CAD build for the part. Positions are in the model's coordinates, mm. Round coordinates to 2 decimals unless told otherwise and drop trailing zeros. Order: outer loops, then holes, each group sorted by start corner. A loop starts at its lowest first (then second) coordinate and runs counter-clockwise, first axis right, second up. Notation, with made-up numbers: M 76.5,15.25 L 83.5,15.25 A28 ccw 83.5,36.25 Z; hole C -30.5,-13 d3. An arc over 180 degrees is marked long. Put each result on its own line as item: value.
```python
from build123d import *

# Parameters (mm, degrees)
SKETCH_1_W                 = 10.16
SKETCH_1_H                 = 2.5
EXTRUDE_1_DEPTH            = 2.5
EXTRUDE_START              = -5
SKETCH_2_R                 = 0.3
EXTRUDE_2_DEPTH            = 7.5
PATTERN_LINEAR_1_COUNT     = 3
PATTERN_LINEAR_1_PITCH     = 2.54
PATTERN_LINEAR_1_COL_COUNT = 2
PATTERN_LINEAR_1_COL_PITCH = 2.54


with BuildPart() as part:
    # 草图1 → 凸台-拉伸1 (new body)
    with BuildSketch(Plane.XY):
        with Locations((5.08, 1.25)):
            Rectangle(SKETCH_1_W, SKETCH_1_H)
    extrude(amount=EXTRUDE_1_DEPTH)

    # 草图2 → 凸台-拉伸2 (add)
    with BuildSketch(Plane.XY.offset(2.5).offset(EXTRUDE_START)):
        with Locations((3.81, 1.25)):
            Circle(SKETCH_2_R)
    extrude_2 = extrude(amount=EXTRUDE_2_DEPTH)

    # 阵列(线性)1: 凸台-拉伸2 ×3
    with Locations(*[(i * PATTERN_LINEAR_1_PITCH, 0, 0) for i in range(1, PATTERN_LINEAR_1_COUNT)]):
        add(extrude_2)

    # 阵列(线性)1 col: 凸台-拉伸2 ×2
    with Locations(*[(-i * PATTERN_LINEAR_1_COL_PITCH, 0, 0) for i in range(1, PATTERN_LINEAR_1_COL_COUNT)]):
        add(extrude_2)


solid = part.part
```
Item 1: Band-saw the part on C-C on y = 1.8. Give the cut face in (x, z).
Answers below:
outline: M 0,0 L 10.16,0 L 10.16,2.5 L 0,2.5 Z
Item 2: Mould opens along Z. For faces 1 (the flat face through (5, 0, 1)), 2 (the flat face through (5, 1, 2.5)), 3 (the flat face through (5, 1, 0)) say: pulls with the +Z half, pulls with the -Z half, needs draft (parallel to the pull), parting line crosses it, or undercut.
Answers below:
face 1: needs draft
face 2: pulls with the +Z half
face 3: pulls with the -Z half
Item 3: Band-saw the part on B-B on z = 3.75. Give the cut face in (x, y), and give its area (3 significant figures).
Answers below:
outline: C 1.27,1.25 d0.6; C 3.81,1.25 d0.6; C 6.35,1.25 d0.6; C 8.89,1.25 d0.6
area: 1.13 mm²
Item 4: Band-saw the part on A-A on x = 8.89. Give the cut face in (y, z).
Answers below:
outline: M 0,0 L 0.95,0 L 0.95,-2.5 L 1.55,-2.5 L 1.55,0 L 2.5,0 L 2.5,2.5 L 1.55,2.5 L 1.55,5 L 0.95,5 L 0.95,2.5 L 0,2.5 Z
Item 5: Probe line 1 along X through (y, z) = (1.15, -1.5); line 2 along X through (y, z) = (1.05, 3); line 3 along Z through (x, y) = (3.5, 1). List the from-to ranges inside material, lowest first. Write a range as [from, to].
Answers below:
line 1: [0.99, 1.55], [3.53, 4.09], [6.07, 6.63], [8.61, 9.17]
line 2: [1.05, 1.49], [3.59, 4.03], [6.13, 6.57], [8.67, 9.11]
line 3: [0, 2.5]
